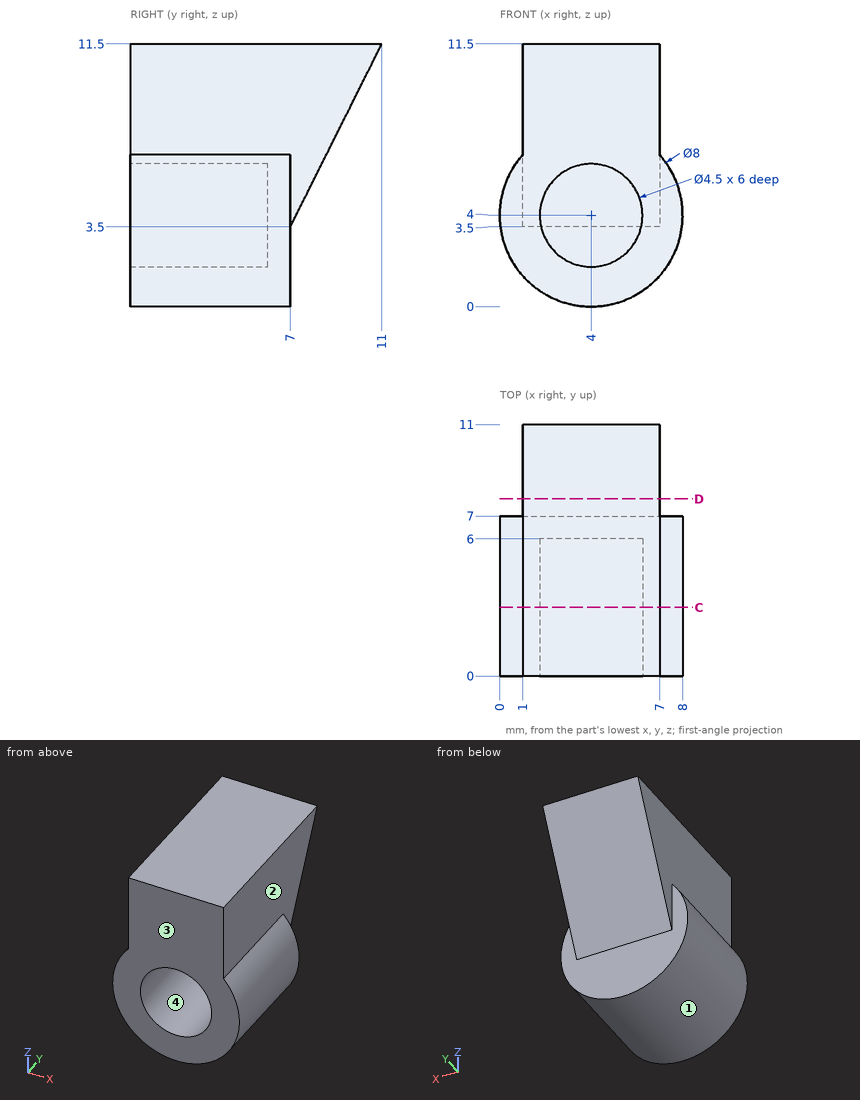
Can you work these out from the drawing? Everything is in mm from the part's minimum corner. Round coordinates to 2 decimals unless told otherwise and drop trailing zeros. Loops run counter-clockwise (first coordinate to the right, second up) from the corner with the lowest first, then second, coordinate; pieces in that order, holes last. Notation, with made-up numbers: (24.5, 35.5) - (76.5, 35.5) arc R36 cw to (76.5, 71.5) - close; hole circle Ø10 at (5.5, 53). An arc over 180 degrees is marked (long way). Answer as CSV lines item,"result".
1. We'd pull the mould along X, two halves only. Please class the marked faces 1, 2, 3 and 4: +X half, -X half, draft (parallel to the pull), parting line (faces both ways), or undercut.
Filled in:
face 1,"parting line"
face 2,"+X half"
face 3,"draft"
face 4,"undercut"
2. For pin 1 Ø3 at (x, z) = (4.5, 9.5) entering from +Y; pin 2 Ø2.5 at (y, z) = (5, 7) entering from +X; pin 3 Ø4 at (y, z) = (4, 7) entering from +X, each with a flat end and sliding along its axis, tell me the tip position at first contact or that it passes through.
Filled in:
pin 1,"stops at y = 10.75"
pin 2,"stops at x = 7.6"
pin 3,"stops at x = 7.87"
3. I want a section at C-C on y = 3. List the corners of the cut face in (x, z) for me, then the cut area to 3 significant figures.
Filled in:
outline,"(1, 6.65) arc R4 ccw (long way) to (7, 6.65) - (7, 11.5) - (1, 11.5) - close; hole circle Ø4.5 at (4, 4)"
area,"57.9 mm^2"
4. Please list where these lines run through material, in increasing order: line 1 along X through (y, z) = (4.75, 4); line 2 along Z through (x, y) = (4, 3.3); line 3 along X through (y, z) = (4.25, 9.75). Write a range as [from, to].
Filled in:
line 1,"x = [0, 1.75], [6.25, 8]"
line 2,"z = [0, 1.75], [6.25, 11.5]"
line 3,"x = [1, 7]"
5. I want a section at D-D on y = 7.75. List the corners of the cut face in (x, z) for me.
Filled in:
outline,"(1, 5) - (7, 5) - (7, 11.5) - (1, 11.5) - close"
